Source: CAD feature listing. Evaluate the final solid. Frame: model axes, mm. Round coordinates to 2 decimals unless told otherwise and drop trailing zeros. Loops run counter-clockwise (first coordinate to the right, second up) from the corner with the lowest first, then second, coordinate; pieces in that order, holes last. Notation, with made-up numbers: M 65.25,26 L 78.25,26 A6 ccw 78.25,30 Z; hole C 30,85.5 d11. An arc over 180 degrees is marked long. Answer as a JSON object with one key per item and string values.
Autodesk Inventor part; units mm, degrees
ref_plane "YZ Plane" through (0, 0, 0) normal (1, 0, 0) x (0, 1, 0)
ref_plane "XZ Plane" through (0, 0, 0) normal (0, 1, 0) x (-1, 0, 0)
ref_plane "XY Plane" through (0, 0, 0) normal (0, 0, 1) x (1, 0, 0)
sketch "Sketch1" plane through (0, 0, 0) normal (0, 0, 1) x (1, 0, 0)
  line L0 (-16, 12.5) -> (-13, 12.5)
  line L1 (-13, 12.5) -> (-13, -9.5)
  line L2 (-13, -9.5) -> (13, -9.5)
  line L3 (13, -9.5) -> (13, 12.9)
  line L4 (13, 12.9) -> (16, 12.9)
  line L5 (16, 12.9) -> (16, -12.5)
  line L6 (16, -12.5) -> (-16, -12.5)
  line L7 (-16, -12.5) -> (-16, 12.5)
  point P0 (0, 0)
  dimension "d0" = 3
  dimension "d2" = 3
  dimension "d3" = 25
  dimension "d4" = 32
  dimension "d5" = 16
  dimension "d7" = 12.5
  dimension "d8" = 3
extrude "Extrusion1" add sketch "Sketch1" against normal blind 457.2
sketch "Sketch10" plane through (-16, -12.5, 0) normal (0, -1, 0) x (1, 0, 0)
  line L0 (32, 0) -> (0, 0)
  line L1 (0, 0) -> (0, -457.2)
  line L2 (32, -457.2) -> (0, -457.2)
  circle A0 centre (16, -12.5) radius 3.175
  circle A1 centre (16, -444.7) radius 3.175
  point P0 (16, 0)
  dimension "d34" = 6.35
  dimension "d35" = 12.5
  dimension "d36" = 12.5
  dimension "d37" = 16
  dimension "d38" = 6.35
hole "Hole1" at (0, -12.5, -444.7) at (0, -12.5, -12.5) direction (0, 1, 0) diameter 6.35 depth 3 tip angle 118
equation "\"d2\" = d0"
equation "\"d8\" = d0"
equation "\"d36\" = d35"
properties part number "18in C-Channel Front" material "Aluminum 6061"
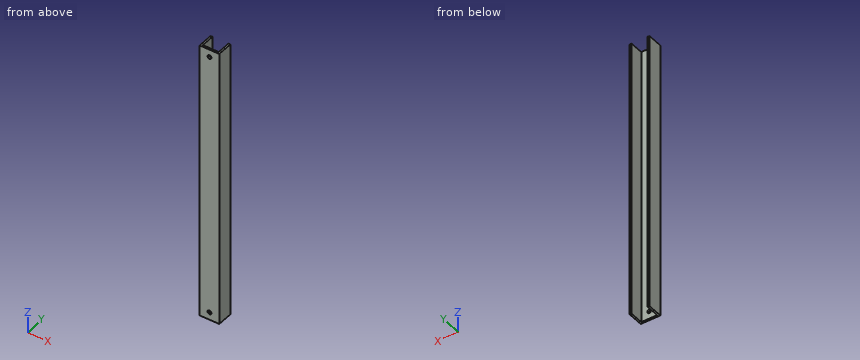
Item 1: Contact query for flat-ended pins moving along their axis: pin 1 Ø8 at (x, z) = (11, -82.5) entering from +Y; pin 2 Ø7.5 at (x, z) = (0, -12.5) entering from +Y; pin 3 Ø5.5 at (x, z) = (0, -444.7) entering from +Y; pin 4 Ø2.5 at (x, z) = (-14.5, -128) entering from +Y. Output: stop coordinate, or through.
Answer sheet:
{"pin 1": "stops at y = 12.9", "pin 2": "stops at y = -9.5", "pin 3": "passes through", "pin 4": "stops at y = 12.5"}
Item 2: Section A-A on y = 1. Return the cut outline in (x, z).
Answer sheet:
{"outline": "M -16,-457.2 L -13,-457.2 L -13,0 L -16,0 Z; M 13,-457.2 L 16,-457.2 L 16,0 L 13,0 Z"}
Item 3: Line query: probe 1 along Z at (x, y) = (0, -11.7) (3 decimals); probe 2 along X at (y, z) = (-3, -398); probe 3 along X at (y, z) = (-11.4, -12.5) (3 decimals). Output: solid intervals per line, ascending. Write a range as from..to.
Answer sheet:
{"probe 1": "z = -457.2..-447.875, -441.525..-15.675, -9.325..0", "probe 2": "x = -16..-13, 13..16", "probe 3": "x = -16..-3.175, 3.175..16"}
Item 4: Section B-B on z = -422. Return the cut outline in (x, y).
Answer sheet:
{"outline": "M -16,-12.5 L 16,-12.5 L 16,12.9 L 13,12.9 L 13,-9.5 L -13,-9.5 L -13,12.5 L -16,12.5 Z"}
Item 5: Section C-C on x = 7. Return the cut outline in (y, z).
Answer sheet:
{"outline": "M -12.5,-457.2 L -9.5,-457.2 L -9.5,0 L -12.5,0 Z"}
